```python
from build123d import *

# Parameters (mm, degrees)
SKETCH1_R           = 25.4
SKETCH1_R_2         = 24
BOSS_EXTRUDE1_DEPTH = 19.05
SKETCH3_R           = 24.7
CUT_EXTRUDE1_DEPTH  = 1.75
SKETCH4_W           = 203.2
SKETCH4_H           = 63.5
SKETCH4_R           = 12.5
BOSS_EXTRUDE2_DEPTH = 3.175


with BuildPart() as part:
    # Sketch1 → Boss-Extrude1 (new body)
    with BuildSketch(Plane(origin=(0, 0, 0), x_dir=(1, 0, 0), z_dir=(0, 1, 0))):
        Circle(SKETCH1_R)
        Circle(SKETCH1_R_2, mode=Mode.SUBTRACT)
    extrude(amount=BOSS_EXTRUDE1_DEPTH)

    # Sketch3 → Cut-Extrude1 (cut)
    with BuildSketch(Plane(origin=(0, 6.35, 0), x_dir=(-1, 0, 0), z_dir=(0, -1, 0))):
        Circle(SKETCH3_R)
    extrude(amount=CUT_EXTRUDE1_DEPTH, mode=Mode.SUBTRACT)

    # Sketch4 → Boss-Extrude2 (add)
    with BuildSketch(Plane(origin=(0, 19.05, 0), x_dir=(1, 0, 0), z_dir=(0, 1, 0))):
        Rectangle(SKETCH4_W, SKETCH4_H)
        Circle(SKETCH4_R, mode=Mode.SUBTRACT)
    extrude(amount=BOSS_EXTRUDE2_DEPTH)


solid = part.part
```
Here's how the part is built. I have some questions about the finished solid (model axes, mm). A direction names the side the tool comes from. Give positions to 0.01 mm unless a question says otherwise; leave off trailing zeros. Loops run counter-clockwise (first coordinate to the right, second up) from the corner with the lowest first, then second, coordinate; pieces in that order, holes last. Notation, with made-up numbers: M -9,-35.5 L 45,-35.5 A21 cw 45,-5.5 Z; hole C 21.5,6.25 d9. An arc over 180 degrees is marked long. Put each result on its own line as item: value. Start each with the question number.
(1) I need wall thicknesses on line 1 along X through (y, z) = (1.9, 0); line 2 along X through (y, z) = (5.35, 0). Which ranges of each line are inside material? Lowest first, please. Write a range as [from, to].
(2) I want a section at A-A on x = 0. Please give me the cut outline in (y, z) (3 decimals).
(3) I want a section at B-B on z = 0. Please give me the cut outline in (x, y) (3 decimals).
(4) I want a section at D-D on x = -66. Please give me the cut outline in (y, z) (3 decimals), then the cut area to 3 significant figures.
(5) For faces 5 (the cylindrical face through (11.923, 20.615, -3.755)), 6 (the cylindrical face through (-23.977, 12.611, -1.055)), 7 (the cylindrical face through (-23.56, 5.49, -7.42)), which set-ups out of +Z, -Z, +X, -X, +Y, -Y let a thin tool reach every point of the face, with its end or its side?
(6) Will these pins go through, and if not, where does the flat tip stop? pin 1 Ø24.5 at (x, z) = (8, -9.5) entering from -Y; pin 2 Ø3 at (y, z) = (14, 19) entering from -X; pin 3 Ø8 at (y, z) = (5.5, -22) entering from +X; pin 4 Ø5 at (y, z) = (16, 5) entering from -X.
(7) If we mould it in two halves opening along X, with no side actions, what happens to faces 1 (the cylindrical face through (-5.506, 9.392, 24.796)), 2 (the flat face through (4, 4.6, -24)), 3 (the cylindrical face through (-23.977, 2.268, -1.055)), 4 (the flat face through (-1, 22.225, -15))? For each: +X half, -X half, draft (parallel to the pull), parting line (faces both ways), or undercut.
(8) I want a section at C-C on z = 19. Please give me the cut outline in (x, y) (3 decimals), then the cut area to 3 significant figures.
Answer block:
1. line 1: [-25.4, -24], [24, 25.4]
1. line 2: [-25.4, -24.7], [24.7, 25.4]
2. outline: M 0,-25.4 L 19.05,-25.4 L 19.05,-31.75 L 22.225,-31.75 L 22.225,-12.5 L 19.05,-12.5 L 19.05,-24 L 6.35,-24 L 6.35,-24.7 L 4.6,-24.7 L 4.6,-24 L 0,-24 Z; M 0,24 L 4.6,24 L 4.6,24.7 L 6.35,24.7 L 6.35,24 L 19.05,24 L 19.05,12.5 L 22.225,12.5 L 22.225,31.75 L 19.05,31.75 L 19.05,25.4 L 0,25.4 Z
3. outline: M -101.6,19.05 L -25.4,19.05 L -25.4,0 L -24,0 L -24,4.6 L -24.7,4.6 L -24.7,6.35 L -24,6.35 L -24,19.05 L -12.5,19.05 L -12.5,22.225 L -101.6,22.225 Z; M 12.5,19.05 L 24,19.05 L 24,6.35 L 24.7,6.35 L 24.7,4.6 L 24,4.6 L 24,0 L 25.4,0 L 25.4,19.05 L 101.6,19.05 L 101.6,22.225 L 12.5,22.225 Z
4. outline: M 19.05,-31.75 L 22.225,-31.75 L 22.225,31.75 L 19.05,31.75 Z
4. area: 202 mm^2
5. face 5: +Y, -Y
5. face 6: -Y
5. face 7: none
6. pin 1: y = 0
6. pin 2: x = -18.41
6. pin 3: x = 17.92
6. pin 4: x = -25.28
7. face 1: parting line
7. face 2: undercut
7. face 3: undercut
7. face 4: draft
8. outline: M -101.6,19.05 L -16.857,19.05 L -16.857,0 L -14.663,0 L -14.663,4.6 L -15.783,4.6 L -15.783,6.35 L -14.663,6.35 L -14.663,19.05 L 14.663,19.05 L 14.663,6.35 L 15.783,6.35 L 15.783,4.6 L 14.663,4.6 L 14.663,0 L 16.857,0 L 16.857,19.05 L 101.6,19.05 L 101.6,22.225 L -101.6,22.225 Z
8. area: 725 mm^2
